Autodesk Inventor part; units mm, degrees
ref_plane "YZ Plane" through (0, 0, 0) normal (1, 0, 0) x (0, 1, 0)
ref_plane "XZ Plane" through (0, 0, 0) normal (0, 1, 0) x (-1, 0, 0)
ref_plane "XY Plane" through (0, 0, 0) normal (0, 0, 1) x (1, 0, 0)
sketch "Sketch1" plane through (0, 0, 0) normal (0, 0, 1) x (1, 0, 0)
  line L0 (0, 0) -> (333.375, 0)
  line L1 (333.375, 0) -> (333.375, 304.8)
  line L2 (320.675, 317.5) -> (12.7, 317.5)
  line L3 (0, 304.8) -> (0, 0)
  circle A0 centre (45.72, 45.72) radius 45.72
  circle A1 centre (287.655, 45.72) radius 45.72
  line L4 (166.6875, 0) -> (166.6875, 7.62)
  arc A2 (287.655, 0) -> (45.72, 0) centre (166.6875, -956.3695) ccw
  arc A3 (12.7, 317.5) -> (0, 304.8) centre (12.7, 304.8) ccw
  arc A4 (333.375, 304.8) -> (320.675, 317.5) centre (320.675, 304.8) ccw
  circle A5 centre (45.72, 45.72) radius 2.413
  circle A6 centre (287.655, 45.72) radius 2.413
  circle A7 centre (307.975, 165.1) radius 2.413
  line L5 (25.4, 165.1) -> (307.975, 165.1)
  circle A8 centre (166.6875, 165.1) radius 2.413
  line L6 (45.72, 45.72) -> (113.792, 45.72)
  line L7 (287.655, 45.72) -> (219.583, 45.72)
  line L8 (49.3862, 39.37) -> (53.0523, 45.72)
  line L9 (49.3862, 52.07) -> (53.0523, 45.72)
  line L10 (42.0538, 39.37) -> (49.3862, 39.37)
  line L11 (42.0538, 52.07) -> (49.3862, 52.07)
  line L12 (42.0538, 52.07) -> (38.3877, 45.72)
  line L13 (38.3877, 45.72) -> (42.0538, 39.37)
  line L14 (291.1818, 39.37) -> (294.848, 45.72)
  line L15 (291.1818, 52.07) -> (294.848, 45.72)
  line L16 (283.8495, 39.37) -> (291.1818, 39.37)
  line L17 (283.8495, 52.07) -> (291.1818, 52.07)
  line L18 (283.8495, 52.07) -> (280.1833, 45.72)
  line L19 (280.1833, 45.72) -> (283.8495, 39.37)
  line L20 (42.0538, 52.07) -> (49.3862, 39.37)
  line L21 (42.0538, 39.37) -> (49.3862, 52.07)
  line L22 (113.792, 95.337) -> (113.792, 63.3371)
  line L23 (113.792, 45.72) -> (113.792, 63.3371)
  circle A9 centre (113.792, 79.3371) radius 4.699
  ellipse E0 centre (113.792, 63.3371) end of major axis (113.7846, 65.3371) minor radius 2
  line L24 (219.583, 45.72) -> (219.583, 63.3371)
  ellipse E1 centre (219.583, 63.3371) end of major axis (219.5756, 65.3371) minor radius 2
  line L25 (219.583, 95.3392) -> (219.583, 63.3371)
  circle A10 centre (219.583, 79.3382) radius 4.699
  ellipse E2 centre (235.5574, 128.7087) end of major axis (235.56, 127.3562) minor radius 1.3525
  ellipse E3 centre (203.5575, 128.6472) end of major axis (203.5601, 127.2947) minor radius 1.3525
  ellipse E4 centre (219.583, 95.337) end of major axis (219.5791, 97.337) minor radius 2
  ellipse E5 centre (129.4616, 128.6451) end of major axis (129.4642, 127.2925) minor radius 1.3525
  ellipse E6 centre (97.4617, 128.6451) end of major axis (97.4643, 127.2925) minor radius 1.3525
  ellipse E7 centre (113.792, 95.337) end of major axis (113.7881, 97.337) minor radius 2
  line L26 (25.4, 165.1) -> (25.4, 157.48)
  line L27 (25.4, 157.48) -> (17.78, 157.48)
  line L28 (17.78, 157.48) -> (17.78, 165.1)
  line L29 (17.78, 165.1) -> (17.78, 172.72)
  line L30 (17.78, 172.72) -> (33.02, 172.72)
  line L31 (33.02, 172.72) -> (33.02, 157.48)
  line L32 (33.02, 157.48) -> (25.4, 157.48)
  point P0 (333.375, 317.5)
  point P1 (0, 317.5)
  point P2 (0, 0)
  point P3 (333.375, 45.72)
  point P4 (0, 45.72)
  point P5 (45.3639, 35.0229)
  point P6 (45.3639, 35.0229)
  point P7 (287.655, 45.72)
  point P8 (287.655, 45.72)
  point P9 (49.2468, 52.07)
  point P10 (291.1818, 52.07)
  point P11 (49.7423, 75.4671)
  point P12 (291.1818, 64.77)
  point P13 (45.72, 45.72)
  dimension "d176" = 91.44
  dimension "d177" = 91.44
  dimension "d174" = 333.375
  dimension "d175" = 317.5
  dimension "d178" = 7.62
  dimension "d179" = 12.7
  dimension "d180" = 4.826
  dimension "d181" = 4.826
  dimension "d184" = 25.4
  dimension "d185" = 4.826
  dimension "d186" = 25.4
  dimension "d188" = 4.826
  dimension "d193" = 68.072
  dimension "d194" = 68.072
  dimension "d195" = 165.1
  dimension "d206" = 12.7
  dimension "d207" = 12.7
  dimension "d208" = 12.7
  dimension "d209" = 7.3323
  dimension "d210" = 7.3323
  dimension "d211" = 7.3323
  dimension "d212" = 7.3323
  dimension "d213" = 7.3323
  dimension "d214" = 7.3323
  dimension "d215" = 12.7
  dimension "d216" = 12.7
  dimension "d217" = 12.7
  dimension "d218" = 7.3323
  dimension "d219" = 7.3323
  dimension "d220" = 7.3323
  dimension "d221" = 7.3323
  dimension "d222" = 7.3323
  dimension "d223" = 7.3323
  dimension "d224" = 17.6171
  dimension "d225" = 17.6171
  dimension "d226" = 9.398
  dimension "d227" = 9.398
  dimension "d228" = 31.9999
  dimension "d229" = 33.308
  dimension "d230" = 31.9999
  dimension "d231" = 33.308
  dimension "d232" = 15.6696
  dimension "d233" = 16.0255
  dimension "d234" = 31.9999
  dimension "d235" = 31.9999
  dimension "d236" = 180
  dimension "d237" = 0
  dimension "d258" = 7.62
  dimension "d259" = 7.62
  dimension "d260" = 7.62
  dimension "d261" = 7.62
  dimension "d262" = 15.24
extrude "Extrusion1" add sketch "Sketch1" along normal blind 5.08 contours A0 A2 | E7 | E0 L22 L23 | L23 L22 E0 | E4 | E1 L25 L24 | L24 L25 E1 | L3 A3 L2 A4 L1 A1 A2 A0 | A2 A1 | E2 | E3 | E5 | E6 picked at (16.5244, 31.421) picked at (316.8042, 60.019)
sketch "Sketch8" plane through (0, 0, 5.08) normal (0, 0, 1) x (1, 0, 0)
  line L0 (33.02, 172.72) -> (33.02, 157.48)
  line L1 (33.02, 157.48) -> (33.02, 165.1)
  line L2 (33.02, 165.1) -> (45.72, 165.1)
  line L3 (45.72, 165.1) -> (64.77, 165.1)
  circle A0 centre (64.9, 165.1) radius 1.3589
  circle A1 centre (45.85, 165.1) radius 1.3589
  line L4 (33.02, 165.1) -> (25.273, 165.1)
  line L5 (17.78, 157.48) -> (17.78, 172.72)
  point P0 (0, 0)
  dimension "d263" = 12.7
  dimension "d264" = 19.05
  dimension "d267" = 2.7178
  dimension "d268" = 2.7178
  dimension "d271" = 7.747
extrude "Extrusion8" cut sketch "Sketch8" against normal blind 28.5115
sketch "Sketch7" plane through (0, 0, 5.08) normal (0, 0, 1) x (1, 0, 0)
  line L0 (0, 304.8) -> (0, 45.72)
  line L1 (320.675, 317.5) -> (12.7, 317.5)
  circle A0 centre (33.02, 241.3) radius 2.413
  circle A1 centre (93.0148, 241.3) radius 2.413
  point P0 (0, 0)
  dimension "d243" = 4.826
  dimension "d244" = 4.826
  dimension "d245" = 76.2
  dimension "d246" = 33.02
  dimension "d247" = 59.9948
  dimension "d248" = 76.2
extrude "Extrusion10" cut sketch "Sketch7" against normal through all
sketch "Sketch9" plane through (0, 0, 5.08) normal (0, 0, 1) x (1, 0, 0)
  circle A0 centre (24.765, 135.255) radius 9.525
  line L0 (33.02, 157.48) -> (17.78, 157.48)
  line L1 (0, 304.8) -> (0, 45.72)
  point P0 (0, 0)
  dimension "d276" = 19.05
  dimension "d277" = 12.7
  dimension "d278" = 15.24
extrude "Extrusion11" cut sketch "Sketch9" against normal through all
sketch "Sketch10" plane through (0, 0, 0) normal (0, 0, -1) x (-1, 0, 0)
  line L0 (-190.5, 318.5819) -> (-190.5, 280.4819)
  line L1 (0, 304.8) -> (0, 45.72)
  circle A0 centre (-190.5, 280.4819) radius 3.175
  circle A1 centre (-38.1866, 267.5069) radius 1.7
  line L2 (-190.5, 280.4819) -> (-38.1866, 267.5069)
  line L3 (-190.5, 280.4819) -> (-38.1866, 280.4819)
  line L4 (-38.1866, 280.4819) -> (-38.1866, 267.5069)
  line L5 (-190.5, 280.4819) -> (-51.9643, 215.8816)
  circle A2 centre (-51.9643, 215.8816) radius 2.4291
  point P0 (0, 0)
  dimension "d282" = 38.1
  dimension "d283" = 190.5
  dimension "d284" = 6.35
  dimension "d287" = 4.869
  dimension "d288" = 152.8651
  dimension "d289" = 152.8572
  dimension "d290" = 25
properties part number "FTC Outside Panels" material "Wood (Oak)"
Input: part model. Units: mm. Frame: model coordinates. Coordinates: 2 decimals unless noted, no trailing zeros. Write each loop counter-clockwise with the first axis right and the second up, starting at its lowest first coordinate (ties: lowest second). Pieces come first, ordered by that corner, then holes.
1) Mould query, pull axis Y, two halves, no side actions, for faces 1 (the cylindrical face through (320.34, 13.75, 2.5)), 2 (the flat face through (164, 161, 0)), 3 (the cylindrical face through (118.274, 77.926, 2.504)). Classes: pulls with the +Y half, pulls with the -Y half, needs draft (parallel to the pull), parting line crosses it, or undercut.
2) Material intervals for line 1 along X through (y, z) = (241.3, 2.4) (3 decimals); line 2 along X through (y, z) = (165.1, 2.75) (1 decimal); line 3 along Y through (x, z) = (28, 1.6), sorted ascending.
3) Section C-C on x = 136.5. Output: boundary loops of the cut face in (y, z).
4) Pin query (flat end, axial travel): pin 1 Ø11 at (x, y) = (219.58, 79.34) entering from -Z. Return the tip coordinate at first contact, or that it passes through.
5) Section A-A on z = 3.2. State how many separate pieces and enclosed holes the cut face has, and give its area (3 significant figures).
6) Section B-B on y = 25. Output: boundary loops of the cut face in (x, z).
Check result:
1. face 1: pulls with the -Y half
1. face 2: needs draft
1. face 3: undercut
2. line 1: x = 0 to 30.607, 35.433 to 90.602, 95.428 to 333.375
2. line 2: x = 0 to 17.8, 33 to 44.5, 47.2 to 63.5, 66.3 to 164.3, 169.1 to 305.6, 310.4 to 333.4
2. line 3: y = 3.57 to 126.3, 144.21 to 157.48, 172.72 to 317.5
3. outline: (7.15, 0) - (317.5, 0) - (317.5, 5.08) - (7.15, 5.08) - close
4. pin 1: stops at z = 0
5. separate pieces: 1
5. enclosed holes: 12
5. area: 103,000 mm2
6. outline: (4.96, 0) - (328.41, 0) - (328.41, 5.08) - (4.96, 5.08) - close
